Model file for the job. Use its own axes, mm. A direction names the side the tool comes from. Round coordinates to 2 decimals unless told otherwise and drop trailing zeros. Loops run counter-clockwise (first coordinate to the right, second up) from the corner with the lowest first, then second, coordinate; pieces in that order, holes last. Notation, with made-up numbers: (20.25, -16) - (36.25, -16) arc R31 ccw to (36.25, 11) - close; hole circle Ø8 at (74, 12.25). An arc over 180 degrees is marked (long way). Answer as a JSON object with one key per item and string values.
from build123d import *

# Parameters (mm, degrees)
F1_DEPTH = 600


with BuildPart() as f1:
    # F0 (on Front) → F1 (new body)
    with BuildSketch(Plane.XZ):
        Polygon((-57.0161717128, 0), (-135, 0), (-150.1679810622, -20.4983499457), (-155.6347784559, -27.8863026074), (-165.3359621243, -40.9966998915), (-96.9383139207, -40.9966998915), (-30.3359621243, -40.9966998915), (0, 0), align=None)
        with BuildLine():
            Line((-150.1679810622, -20.4983499457), (-135, 0))
            Line((-135, 0), (-57.0161717128, 0))
            ThreePointArc((-57.0161717128, 0), (-56.9075739834, 61.0124300524), (-116.5067681147, 74.0686344498))
            ThreePointArc((-116.5067681147, 74.0686344498), (-118.6940510107, 72.9068001121), (-120.8193157857, 71.6350630594))
            ThreePointArc((-120.8193157857, 71.6350630594), (-134.2868225707, 58.9282400507), (-142.0255883167, 42.1071641426))
            Line((-142.0255883167, 42.1071641426), (-232.0590932336, 42.1071641426))
            Line((-232.0590932336, 42.1071641426), (-256.4444055904, 9.1523058673))
            Line((-256.4444055904, 9.1523058673), (-234.9909992313, -19.8403088568))
            Line((-234.9909992313, -19.8403088568), (-220.3099429607, 0))
            Line((-220.3099429607, 0), (-176.7144793644, 0))
            Line((-176.7144793644, 0), (-191.8824604265, -20.4983499457))
            Line((-191.8824604265, -20.4983499457), (-150.1679810622, -20.4983499457))
        make_face()
        with BuildLine():
            ThreePointArc((-132.8527878768, 40.9173611322), (-78.7209860622, 66.5720298878), (-61.7161940581, 9.132922604))
            Line((-61.7161940581, 9.132922604), (-82.854176665, 9.132922604))
            Line((-82.854176665, 9.132922604), (-132.8527878768, 40.9173611322))
        make_face(mode=Mode.SUBTRACT)
        Polygon((20.9851757958, 28.3598374347), (0, 0), (-30.3359621243, -40.9966998915), (-71.6739757792, -96.8618190849), (-65.4539629325, -105.2676840103), (106.5884042597, 127.2342312906), (94.1483785662, 127.2342312906), align=None)
        with BuildLine():
            ThreePointArc((-120.8193157857, 71.6350630594), (-118.6940510107, 72.9068001121), (-116.5067681147, 74.0686344498))
            Line((-116.5067681147, 74.0686344498), (-122.841415611, 83.044531927))
            ThreePointArc((-122.841415611, 83.044531927), (-124.6735165199, 81.3559804602), (-126.9215099137, 80.2815850499))
            Line((-126.9215099137, 80.2815850499), (-120.8193157857, 71.6350630594))
        make_face()
        Polygon((-165.3359621243, -40.9966998915), (-155.6347784559, -27.8863026074), (-197.0568264004, -27.8863026074), (-207.4885144694, -41.9839199295), (-167.8028032048, -41.9839199295), (-173.6653593057, -49.906709788), (-213.9235590781, -49.906709788), (-227.7684772045, -68.6170427956), (-195.4038739204, -68.6170427956), (-177.2415726766, -68.6170427956), (-168.0213273478, -68.6170427956), (-202.9398083687, -115.8066615462), (-275.9852580547, -115.8066615462), (-248.7127541929, -152.6633352041), (-179.5672774315, -152.6633352041), (-96.9383139207, -40.9966998915), align=None)
        with BuildLine():
            Line((-22.2512632608, 28.3598374347), (20.9851757958, 28.3598374347))
            Line((20.9851757958, 28.3598374347), (94.1483785662, 127.2342312906))
            Line((94.1483785662, 127.2342312906), (-75.7271274924, 127.2342312906))
            Line((-75.7271274924, 127.2342312906), (-91.8894008887, 105.3921723746))
            ThreePointArc((-91.8894008887, 105.3921723746), (-37.6565854676, 84.4262603806), (-22.2512632608, 28.3598374347))
        make_face()
        with BuildLine():
            ThreePointArc((-126.9215099137, 80.2815850499), (-124.6735165199, 81.3559804602), (-122.841415611, 83.044531927))
            ThreePointArc((-122.841415611, 83.044531927), (-121.4714983754, 85.5077083569), (-120.9969189392, 88.285960634))
            ThreePointArc((-120.9969189392, 88.285960634), (-136.093489638, 93.26518765), (-126.9215099137, 80.2815850499))
        make_face()
        Polygon((-65.4539629325, -105.2676840103), (-71.6739757792, -96.8618190849), (-98.7022470538, -133.3884313442), (-92.4822342071, -141.7942962696), align=None)
        Polygon((-98.7022470538, -133.3884313442), (-71.6739757792, -96.8618190849), (-82.7770473941, -81.8568789745), (-116.2240564073, -81.8568789745), (-141.3440536534, -115.804606894), (-111.7135926971, -115.804606894), align=None)
        Polygon((-92.4822342071, -141.7942962696), (-98.7022470538, -133.3884313442), (-144.5443985877, -195.3405435308), (-137.2889383083, -202.3470815625), align=None)
        Polygon((-41.0452445793, -138.2541736742), (-65.4539629325, -105.2676840103), (-92.4822342071, -141.7942962696), (-68.0735158539, -174.7807859336), align=None)
        Polygon((-177.2415726766, -68.6170427956), (-195.4038739204, -68.6170427956), (-186.1869692802, -80.7060524821), align=None)
    extrude(amount=F1_DEPTH)


solid = f1.part
1) Slice it at C-C on x = 45. List the corners of the cut face in (y, z), then the cut area to 3 significant figures.
Values follow:
{"outline": "(-600, 44) - (0, 44) - (0, 127.23) - (-600, 127.23) - close", "area": "49,900 mm²"}
2) Slice it at A-A on z = -165.5. List the corners of the cut face in (x, y).
Values follow:
{"outline": "(-122.46, -600) - (-110.02, -600) - (-110.02, 0) - (-122.46, 0) - close; (-74.94, -600) - (-61.21, -600) - (-61.21, 0) - (-74.94, 0) - close"}
3) Tool access for faces 4 (the flat face through (-199, -296, 0)), 5 (the flat face through (-245.9, -295.8, -5.1)): list every direction of +Z, -Z, +X, -X, +Y, -Y with a clear straight run to the whole face (end or side of a thin tool).
Values follow:
{"face 4": "+Y, -Y", "face 5": "-X, +Y, -Y"}
4) Drop flat-ended pins along their axis: P1, Ø12, axis at x = -197, y = -425, coming from the -Z side; P2, Ø10, axis at x = -106, y = -407, coming from the +Z side; P3, Ø5, axis at x = -85.5, z = 12.5, coming from the +Y side; P4, Ø3, axis at x = -30, y = -220, coming from the -Z side. Give the stop position or say it passes through.
Values follow:
{"P1": "z = -152.66", "P2": "z = 78.79", "P3": "y = 0", "P4": "z = -59.38"}
5) Two-plate mould, pull along Z, no slides. Class faces 1 (the flat face through (-194, -296, -49.907)), 2 (the flat face through (-80.449, -295.8, -158.057)), 3 (the flat face through (-83.695, -295.8, 116.466)): pulls with the +Z half, pulls with the -Z half, needs draft (parallel to the pull), parting line crosses it, or undercut.
Values follow:
{"face 1": "undercut", "face 2": "pulls with the -Z half", "face 3": "pulls with the +Z half"}
6) Slice it at B-B on z = -58. List the corners of the cut face in (x, y).
Values follow:
{"outline": "(-219.91, -600) - (-109.52, -600) - (-109.52, 0) - (-219.91, 0) - close; (-42.92, -600) - (-30.48, -600) - (-30.48, 0) - (-42.92, 0) - close"}
7) Probe probe 1 along Z at (x, y) = (-213, -463); probe 2 along Z at (x, y) = (-214, -218); probe 3 along Z at (x, y) = (-195, -523.5). List the from-to ranges inside material, lowest first.
Values follow:
{"probe 1": "-152.66 to -115.81, -68.62 to -49.91, 0 to 42.11", "probe 2": "-152.66 to -115.81, -68.62 to -50.01, 0 to 42.11", "probe 3": "-152.66 to -105.08, -69.15 to -49.91, -41.98 to -27.89, 0 to 42.11"}
